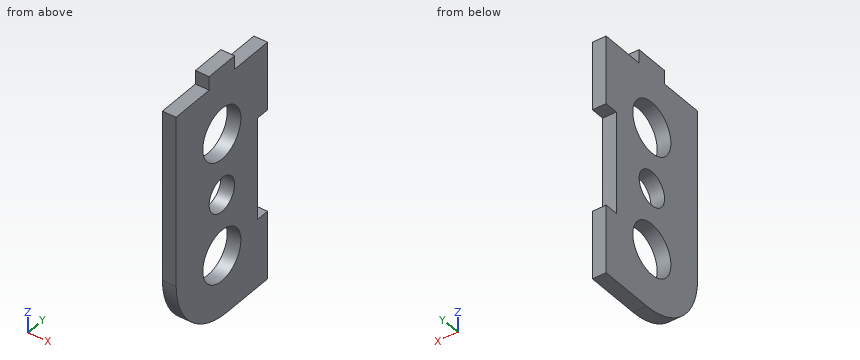
from build123d import *

# Parameters (mm, degrees)
AUFSATZ_LINEAR_AUSTRAGEN1_DEPTH = 4
SKIZZE3_W                       = 30
SKIZZE3_H                       = 4
SCHNITT_LINEAR_AUSTRAGEN2_DEPTH = 77.26270386
VERRUNDUNG1_R                   = 20
SKIZZE5_R                       = 7.5
SKIZZE5_R_2                     = 5
SCHNITT_LINEAR_AUSTRAGEN4_DEPTH = 77.26270386


with BuildPart() as part:
    # Skizze1 → Aufsatz-Linear austragen1 (new body)
    with BuildSketch(Plane(origin=(0, 0, 0), x_dir=(0, 0, -1), z_dir=(1, 0, 0))):
        Polygon((0, -5), (0, 5), (4, 5), (4, 18), (74, 18), (74, -18), (4, -18), (4, -5), align=None)
    extrude(amount=AUFSATZ_LINEAR_AUSTRAGEN1_DEPTH)

    # Skizze3 → Schnitt-Linear austragen2 (cut, through all)
    with BuildSketch(Plane(origin=(4, 0, 0), x_dir=(0, 0, -1), z_dir=(1, 0, 0))):
        with Locations((39, 16)):
            Rectangle(SKIZZE3_W, SKIZZE3_H)
    extrude(amount=-SCHNITT_LINEAR_AUSTRAGEN2_DEPTH, mode=Mode.SUBTRACT)

    # Verrundung1
    verrundung1_edges = [part.edges().sort_by_distance(p)[0] for p in [
        (2, -18, -74),
    ]]
    fillet(verrundung1_edges, radius=VERRUNDUNG1_R)

    # Skizze5 → Schnitt-Linear austragen4 (cut, through all)
    with BuildSketch(Plane(origin=(4, 0, 0), x_dir=(0, 0, -1), z_dir=(1, 0, 0))):
        with Locations((20, 0)):
            Circle(SKIZZE5_R)
        with Locations((56, 0)):
            Circle(SKIZZE5_R)
        with Locations((38, 0)):
            Circle(SKIZZE5_R_2)
    extrude(amount=-SCHNITT_LINEAR_AUSTRAGEN4_DEPTH, mode=Mode.SUBTRACT)


solid = part.part
Work out the finished part from the listing and answer in its coordinate system (mm). Round coordinates to 2 decimals unless told otherwise and drop trailing zeros. Order: outer loops, then holes, each group sorted by start corner. A loop starts at its lowest first (then second) coordinate and runs counter-clockwise, first axis right, second up. Notation, with made-up numbers: M -15.5,69.5 L 17.5,69.5 A17 cw 17.5,85.5 Z; hole C 79,54.25 d8. An arc over 180 degrees is marked long. Put each result on its own line as item: value. Start each with the question number.
Q1. Section A-A, the plane z = -20 is taken. Write down the section's boundary in (x, y), and give its area (3 significant figures).
Q2. Section B-B, the plane x = 0.75 is taken. Write down the section's boundary in (y, z).
Q3. Straight lines are drawn through the part: L1, parallel to Z at x = 3.45, y = 16; L2, parallel to Y at x = 3.25, z = -19.5; L3, parallel to Z at x = 0.2, y = -2. For each, find the intervals that lie inside material, in ascending order. Write a range as [from, to].
Q4. Section C-C, the plane y = -6 is taken. Write down the section's boundary in (x, z).
Q5. Section D-D, the plane z = -38 is taken. Write down the section's boundary in (x, y), and give its area (3 significant figures).
Q6. Flat-ended cylindrical pins translate along their axes: pin 1 (1.2 mm diameter, centred on x = 1.5, z = -2, fed in from +Y); pin 2 (2 mm diameter, centred on x = 2, z = -64, fed in from -Y); pin 3 (2 mm diameter, centred on x = 1.5, z = -34, fed in from +Y). Find the tip coordinate at first contact, or state that the pin passes through.
Findings below:
1. outline: M 0,-18 L 4,-18 L 4,-7.5 L 0,-7.5 Z; M 0,7.5 L 4,7.5 L 4,18 L 0,18 Z
1. area: 84.0 mm^2
2. outline: M -18,-54 A20 ccw 2,-74 L 18,-74 L 18,-54 L 14,-54 L 14,-24 L 18,-24 L 18,-4 L 5,-4 L 5,0 L -5,0 L -5,-4 L -18,-4 Z; hole C 0,-56 d15; hole C 0,-20 d15; hole C 0,-38 d10
3. L1: z = [-74, -54], [-24, -4]
3. L2: y = [-18, -7.48], [7.48, 18]
3. L3: z = [-73.6, -63.23], [-48.77, -42.58], [-33.42, -27.23], [-12.77, 0]
4. outline: M 0,-72.33 L 4,-72.33 L 4,-60.5 L 0,-60.5 Z; M 0,-51.5 L 4,-51.5 L 4,-24.5 L 0,-24.5 Z; M 0,-15.5 L 4,-15.5 L 4,-4 L 0,-4 Z
5. outline: M 0,-18 L 4,-18 L 4,-5 L 0,-5 Z; M 0,5 L 4,5 L 4,14 L 0,14 Z
5. area: 88.0 mm^2
6. pin 1: stops at y = 5
6. pin 2: stops at y = -15.86
6. pin 3: stops at y = 14
